from build123d import *

# Parameters (mm, degrees)
F0_W     = 101.6
F0_H     = 50.8
F1_DEPTH = 127
F2_R     = 32.820623
F3_DEPTH = 120.243898
F4_R     = 19.05
F5_SIZE2 = 10.16
F5_SIZE  = 10.16


with BuildPart() as f1:
    # F0 (on Top) → F1 (new body)
    with BuildSketch(Plane.XY):
        with Locations((50.8, 25.4)):
            Rectangle(F0_W, F0_H)
    extrude(amount=F1_DEPTH)

    # F2 (on face) → F3 (cut)
    with BuildSketch(Plane.XZ):
        with Locations((54.029975, 60.365319)):
            Circle(F2_R)
    extrude(amount=-F3_DEPTH, mode=Mode.SUBTRACT)

    # F4
    f4_edges = [f1.edges().sort_by_distance(p)[0] for p in [
        (101.6, 25.4, 127),
        (0, 25.4, 127),
        (101.6, 25.4, 0),
        (0, 25.4, 0),
    ]]
    fillet(f4_edges, radius=F4_R)

    # F5
    f5_edges = [f1.edges().sort_by_distance(p)[0] for p in [
        (101.6, 0, 63.5),
        (0, 50.8, 63.5),
    ]]
    chamfer(f5_edges, length=F5_SIZE, length2=F5_SIZE2)


solid = f1.part
For this review, take the finished solid that the model builds, in its own axes (mm). Round coordinates to 2 decimals unless told otherwise and drop trailing zeros. Order: outer loops, then holes, each group sorted by start corner. A loop starts at its lowest first (then second) coordinate and runs counter-clockwise, first axis right, second up. Notation, with made-up numbers: (28.25, 29.5) -> (44.25, 29.5) arc R26 cw to (44.25, 64.5) -> close; hole circle Ø4 at (9.5, -23). An arc over 180 degrees is marked (long way). Write item = value, one per line. Start each with the question number.
1) Take a section at C-C on x = 79.5. State the section outline as (y, z) points, plus the area to 3 significant figures.
2) To check wall thickness, follow line 1 (X direction, y = 34, z = 60.5); line 2 (X direction, y = 34, z = 58); line 3 (Z direction, x = 43, y = 19). State the ranges of each line that lie inside material, in increasing order. Write a range as from..to.
3) Insertion check: pin 1 (5 mm diameter, centred on x = 61.5, z = 88.5, fed in from -Y); pin 2 (4 mm diameter, centred on x = 89, y = 17, fed in from +Z). Each pin has a flat end and moves straight along its axis. Give the tip position at first contact, or say it passes through.
4) Take a section at D-D on z = 104. State the section outline as (x, y) points.
5) Take a section at B-B on y = 6.5. State the section outline as (x, z) points.
6) Take a section at A-A on z = 52. State the section outline as (x, y) points, plus the area to 3 significant figures.
Verdict:
q1.outline = (0, 10.16) -> (10.16, 0) -> (40.64, 0) -> (50.8, 10.16) -> (50.8, 39.67) -> (0, 39.67) -> close; (0, 81.06) -> (50.8, 81.06) -> (50.8, 116.84) -> (40.64, 127) -> (10.16, 127) -> (0, 116.84) -> close
q1.area = 4,140 mm2
q2.line_1 = 0..21.21, 86.85..101.6
q2.line_2 = 0..21.29, 86.77..101.6
q2.line_3 = 0..29.45, 91.28..127
q3.pin_1 = through
q3.pin_2 = 126.47
q4.outline = (0, 10.16) -> (10.16, 0) -> (91.44, 0) -> (101.6, 10.16) -> (101.6, 40.64) -> (91.44, 50.8) -> (10.16, 50.8) -> (0, 40.64) -> close
q5.outline = (3.66, 19.05) arc R15.39 ccw to (19.05, 3.66) -> (82.55, 3.66) arc R15.39 ccw to (97.94, 19.05) -> (97.94, 107.95) arc R15.39 ccw to (82.55, 123.34) -> (19.05, 123.34) arc R15.39 ccw to (3.66, 107.95) -> close; hole circle Ø65.64 at (54.03, 60.37)
q6.outline = (0, 10.16) -> (10.16, 0) -> (22.29, 0) -> (22.29, 50.8) -> (10.16, 50.8) -> (0, 40.64) -> close; (85.77, 0) -> (91.44, 0) -> (101.6, 10.16) -> (101.6, 40.64) -> (91.44, 50.8) -> (85.77, 50.8) -> close
q6.area = 1,730 mm2
